Here's how the part is built. I have some questions about the finished solid (model axes, mm). Coordinates: 2 decimals unless noted, no trailing zeros. Order: outer loops, then holes, each group sorted by start corner. A loop starts at its lowest first (then second) coordinate and runs counter-clockwise, first axis right, second up.
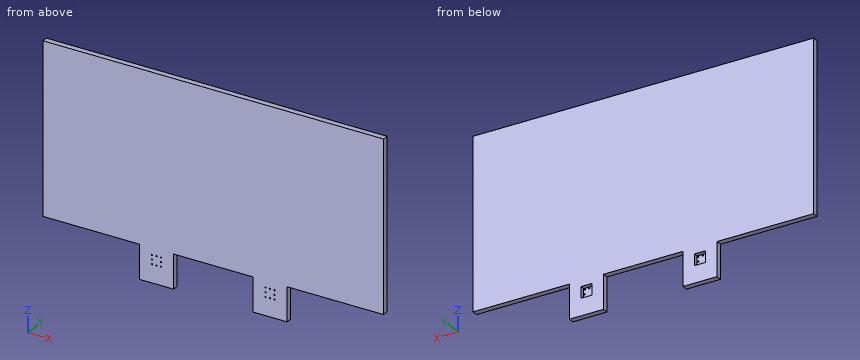
```python
from build123d import *

# Parameters (mm, degrees)
EXTRUDE_1_DEPTH     = 10
SKETCH_2_W          = 20
SKETCH_2_H          = 20
SKETCH_2_R          = 1.05
CUT_EXTRUDE_1_DEPTH = 8
SKETCH_2_4_R        = 1.05
CUT_EXTRUDE_3_DEPTH = 367.33318168


with BuildPart() as part:
    # Sketch 1 → Extrude 1 (new body)
    with BuildSketch(Plane(origin=(0, 0, 0), x_dir=(1, 0, 0), z_dir=(0, 1, 0))):
        Polygon((-300, -150), (300, -150), (300, 150), (130, 150), (130, 210), (70, 210), (70, 150), (-70, 150), (-70, 210), (-130, 210), (-130, 150), (-300, 150), align=None)
    extrude(amount=EXTRUDE_1_DEPTH)

    # Sketch 2 → Cut-Extrude 1 (cut)
    # profile 1 of 2: a face of its own
    with BuildSketch(Plane(origin=(0, 10, 0), x_dir=(1, 0, 0), z_dir=(0, 1, 0))):
        with Locations((-100, 170)):
            Rectangle(SKETCH_2_W, SKETCH_2_H)
        with Locations(Location((-108, 178, 0), (0, 0, 270))):
            Circle(SKETCH_2_R, mode=Mode.SUBTRACT)
        with Locations(Location((-92, 178, 0), (0, 0, 270))):
            Circle(SKETCH_2_R, mode=Mode.SUBTRACT)
        with Locations(Location((-92, 162, 0), (0, 0, 270))):
            Circle(SKETCH_2_R, mode=Mode.SUBTRACT)
        with Locations(Location((-108, 162, 0), (0, 0, 270))):
            Circle(SKETCH_2_R, mode=Mode.SUBTRACT)
        with Locations(Location((-100, 178, 0), (0, 0, 270))):
            Circle(SKETCH_2_R, mode=Mode.SUBTRACT)
        with Locations(Location((-100, 162, 0), (0, 0, 270))):
            Circle(SKETCH_2_R, mode=Mode.SUBTRACT)
        with Locations(Location((-108, 170, 0), (0, 0, 270))):
            Circle(SKETCH_2_R, mode=Mode.SUBTRACT)
        with Locations(Location((-92, 170, 0), (0, 0, 270))):
            Circle(SKETCH_2_R, mode=Mode.SUBTRACT)
    # profile 2 of 2: a face of its own
    with BuildSketch(Plane(origin=(0, 10, 0), x_dir=(1, 0, 0), z_dir=(0, 1, 0))):
        with Locations((100, 170)):
            Rectangle(SKETCH_2_W, SKETCH_2_H)
        with Locations(Location((108, 162, 0), (0, 0, 270))):
            Circle(SKETCH_2_R, mode=Mode.SUBTRACT)
        with Locations(Location((92, 162, 0), (0, 0, 270))):
            Circle(SKETCH_2_R, mode=Mode.SUBTRACT)
        with Locations(Location((92, 178, 0), (0, 0, 270))):
            Circle(SKETCH_2_R, mode=Mode.SUBTRACT)
        with Locations(Location((108, 178, 0), (0, 0, 270))):
            Circle(SKETCH_2_R, mode=Mode.SUBTRACT)
        with Locations(Location((108, 170, 0), (0, 0, 270))):
            Circle(SKETCH_2_R, mode=Mode.SUBTRACT)
        with Locations(Location((100, 162, 0), (0, 0, 270))):
            Circle(SKETCH_2_R, mode=Mode.SUBTRACT)
        with Locations(Location((92, 170, 0), (0, 0, 270))):
            Circle(SKETCH_2_R, mode=Mode.SUBTRACT)
        with Locations(Location((100, 178, 0), (0, 0, 270))):
            Circle(SKETCH_2_R, mode=Mode.SUBTRACT)
    extrude(amount=-CUT_EXTRUDE_1_DEPTH, mode=Mode.SUBTRACT)

    # Sketch 2_4 → Cut-Extrude 3 (cut, through all)
    with BuildSketch(Plane(origin=(0, 10, 0), x_dir=(1, 0, 0), z_dir=(0, 1, 0))):
        with Locations(Location((-92, 170, 0), (0, 0, 270))):
            Circle(SKETCH_2_4_R)
        with Locations(Location((-100, 178, 0), (0, 0, 270))):
            Circle(SKETCH_2_4_R)
        with Locations(Location((-108, 170, 0), (0, 0, 270))):
            Circle(SKETCH_2_4_R)
        with Locations(Location((-100, 162, 0), (0, 0, 270))):
            Circle(SKETCH_2_4_R)
        with Locations(Location((108, 170, 0), (0, 0, 270))):
            Circle(SKETCH_2_4_R)
        with Locations(Location((100, 178, 0), (0, 0, 270))):
            Circle(SKETCH_2_4_R)
        with Locations(Location((92, 170, 0), (0, 0, 270))):
            Circle(SKETCH_2_4_R)
        with Locations(Location((100, 162, 0), (0, 0, 270))):
            Circle(SKETCH_2_4_R)
        with Locations(Location((-108, 178, 0), (0, 0, 270))):
            Circle(SKETCH_2_4_R)
        with Locations(Location((-92, 178, 0), (0, 0, 270))):
            Circle(SKETCH_2_4_R)
        with Locations(Location((-92, 162, 0), (0, 0, 270))):
            Circle(SKETCH_2_4_R)
        with Locations(Location((-108, 162, 0), (0, 0, 270))):
            Circle(SKETCH_2_4_R)
        with Locations(Location((92, 178, 0), (0, 0, 270))):
            Circle(SKETCH_2_4_R)
        with Locations(Location((108, 178, 0), (0, 0, 270))):
            Circle(SKETCH_2_4_R)
        with Locations(Location((108, 162, 0), (0, 0, 270))):
            Circle(SKETCH_2_4_R)
        with Locations(Location((92, 162, 0), (0, 0, 270))):
            Circle(SKETCH_2_4_R)
    extrude(amount=-CUT_EXTRUDE_3_DEPTH, mode=Mode.SUBTRACT)


solid = part.part
```
Q1. If we section it at A-A on y = 6.75: Write out the boundary of the cut face in (x, z).
Q2. I need wall thicknesses on L1, parallel to Z at x = 108, y = 0.8; L2, parallel to X at y = 3, z = -166; L3, parallel to X at y = 0.55, z = -170. Which ranges of each line are inside material? Lowest first, please.
Q3. If we section it at B-B on x = -34: Write out the boundary of the cut face in (y, z).
Q4. Will these pins go through, and if not, where does the flat tip stop? pin 1 (1.3 mm diameter, centred on x = -92, z = -170, fed in from +Y); pin 2 (2.5 mm diameter, centred on x = 108, z = -178, fed in from +Y); pin 3 (3 mm diameter, centred on y = 3.5, z = -195, fed in from +X); pin 4 (4 mm diameter, centred on y = 5, z = -166, fed in from -X).
Reply:
1. outline: (-300, -150) - (-130, -150) - (-130, -210) - (-70, -210) - (-70, -150) - (70, -150) - (70, -210) - (130, -210) - (130, -150) - (300, -150) - (300, 150) - (-300, 150) - close; hole (-110, -180) - (-90, -180) - (-90, -160) - (-110, -160) - close; hole (90, -180) - (110, -180) - (110, -160) - (90, -160) - close
2. L1: z = -210 to -179.05, -176.95 to -171.05, -168.95 to -163.05, -160.95 to 150
2. L2: x = -130 to -110, -90 to -70, 70 to 90, 110 to 130
2. L3: x = -130 to -109.05, -106.95 to -93.05, -90.95 to -70, 70 to 90.95, 93.05 to 106.95, 109.05 to 130
3. outline: (0, -150) - (10, -150) - (10, 150) - (0, 150) - close
4. pin 1: passes through
4. pin 2: stops at y = 2
4. pin 3: stops at x = 130
4. pin 4: stops at x = -130
